```python
from build123d import *
from build123d.topology import SkipClean

# Parameters (mm, degrees)
SKETCH1_W           = 53.05
SKETCH1_H           = 118.2
SKETCH1_W_2         = 45.05
SKETCH1_H_2         = 110.2
BOSS_EXTRUDE1_DEPTH = 60.67
SKETCH2_W           = 53.05
SKETCH2_H           = 118.2
BOSS_EXTRUDE2_DEPTH = 4
SKETCH3_W           = 30
SKETCH3_H           = 22.2
CUT_EXTRUDE1_DEPTH  = 4
SKETCH4_W           = 45
SKETCH4_H           = 38.2
CUT_EXTRUDE2_DEPTH  = 4
SKETCH5_W           = 37.05
SKETCH5_H           = 23
CUT_EXTRUDE3_DEPTH  = 4
SKETCH6_R           = 13.5
SKETCH6_R_2         = 11.5
BOSS_EXTRUDE3_DEPTH = 3.4
SKETCH9_R           = 11.5
CUT_EXTRUDE4_DEPTH  = 5.5
SKETCH10_W          = 1.3
SKETCH10_H          = 30
CUT_EXTRUDE6_DEPTH  = 100.939788873
SKETCH8_R           = 13.5
BOSS_EXTRUDE5_DEPTH = 3
SKETCH12_R          = 3.325
CUT_EXTRUDE8_DEPTH  = 85.508097393


with BuildPart() as part:
    # Sketch1 → Boss-Extrude1 (new body)
    with BuildSketch(Plane.XY):
        Rectangle(SKETCH1_W, SKETCH1_H)
        Rectangle(SKETCH1_W_2, SKETCH1_H_2, mode=Mode.SUBTRACT)
    extrude(amount=BOSS_EXTRUDE1_DEPTH)

    # Sketch2 → Boss-Extrude2 (add)
    with BuildSketch(Plane.XY):
        Rectangle(SKETCH2_W, SKETCH2_H)
    extrude(amount=-BOSS_EXTRUDE2_DEPTH)

    # Sketch3 → Cut-Extrude1 (cut)
    with BuildSketch(Plane(origin=(26.525, 0, 0), x_dir=(0, 0, -1), z_dir=(1, 0, 0))):
        with Locations((-45.67, 0)):
            Rectangle(SKETCH3_W, SKETCH3_H)
    extrude(amount=-CUT_EXTRUDE1_DEPTH, mode=Mode.SUBTRACT)

    # Sketch4 → Cut-Extrude2 (cut)
    with BuildSketch(Plane.ZY.offset(26.525)):
        with Locations((38.17, 0)):
            Rectangle(SKETCH4_W, SKETCH4_H)
    extrude(amount=-CUT_EXTRUDE2_DEPTH, mode=Mode.SUBTRACT)

    # Sketch5 → Cut-Extrude3 (cut)
    with BuildSketch(Plane.XZ.offset(59.1)):
        with Locations((0, 49.17)):
            Rectangle(SKETCH5_W, SKETCH5_H)
    extrude(amount=-CUT_EXTRUDE3_DEPTH, mode=Mode.SUBTRACT)

    # Sketch6 → Boss-Extrude3 (add)
    with BuildSketch(Plane.XY):
        Circle(SKETCH6_R)
        Circle(SKETCH6_R_2, mode=Mode.SUBTRACT)
    extrude(amount=BOSS_EXTRUDE3_DEPTH)

    # Sketch9 → Cut-Extrude4 (cut)
    with SkipClean():  # the faces are left unmerged after this step: merging them gives an invalid solid
        with BuildSketch(Plane(origin=(0, 0, -4), x_dir=(-1, 0, 0), z_dir=(0, 0, -1))):
            Circle(SKETCH9_R)
        extrude(amount=-CUT_EXTRUDE4_DEPTH, mode=Mode.SUBTRACT)
    add(part.part.scale(1), mode=Mode.REPLACE)  # the faces are merged on a copy

    # Sketch10 → Cut-Extrude6 (cut, through all)
    with BuildSketch(Plane(origin=(26.525, 0, 0), x_dir=(0, 0, -1), z_dir=(1, 0, 0))):
        with Locations((3.35, 44.1)):
            Rectangle(SKETCH10_W, SKETCH10_H)
        with Locations((3.35, -44.1)):
            Rectangle(SKETCH10_W, SKETCH10_H)
    extrude(amount=-CUT_EXTRUDE6_DEPTH, mode=Mode.SUBTRACT)

    # Sketch8 → Boss-Extrude5 (add)
    with SkipClean():  # the faces are left unmerged after this step: merging them gives an invalid solid
        with BuildSketch(Plane.XY.offset(3.4)):
            Circle(SKETCH8_R)
        extrude(amount=BOSS_EXTRUDE5_DEPTH)

    # Sketch12 → Cut-Extrude8 (cut, through all)
    with SkipClean():  # the faces are left unmerged after this step: merging them gives an invalid solid
        with BuildSketch(Plane.XY.offset(6.4)):
            Circle(SKETCH12_R)
        extrude(amount=-CUT_EXTRUDE8_DEPTH, mode=Mode.SUBTRACT)


solid = part.part
```
Check sheet for the modelled part. Datum: model origin and axes. Units: mm. A direction names the side the tool comes from. Round coordinates to 2 decimals unless told otherwise and drop trailing zeros. Order: outer loops, then holes, each group sorted by start corner. A loop starts at its lowest first (then second) coordinate and runs counter-clockwise, first axis right, second up. Notation, with made-up numbers: M 84.5,89 L 97.5,89 A28 ccw 97.5,109 Z; hole C 75.5,-39.5 d8. An arc over 180 degrees is marked long. Answer in a Markdown table with one row per item.
(1) Set-up check for faces 1 (the flat face through (18.525, -57, 49)), 2 (the flat face through (25, 0, 30.67)), 3 (the cylindrical face through (-2.93, -13.18, 3.16)): record each of +Z, -Z, +X, -X, +Y, -Y from which the full face is reachable in a straight line by a thin tool's end or side.
Findings:
| item | result |
|---|---|
| face 1 | +Z, -Y |
| face 2 | +Z, +X, -X |
| face 3 | +Z |
(2) Section check B-B on x = 0. Record the boundary of the cut face in (y, z) (3 decimals).
Findings:
| item | result |
|---|---|
| outline | M -59.1,-2.7 L -29.1,-2.7 L -29.1,-4 L -11.5,-4 L -11.5,3.4 L -3.325,3.4 L -3.325,6.4 L -13.5,6.4 L -13.5,0 L -55.1,0 L -55.1,37.67 L -59.1,37.67 Z; M 3.325,3.4 L 11.5,3.4 L 11.5,-4 L 29.1,-4 L 29.1,-2.7 L 59.1,-2.7 L 59.1,60.67 L 55.1,60.67 L 55.1,0 L 13.5,0 L 13.5,6.4 L 3.325,6.4 Z |
(3) Draft check along X on faces 4 (the flat face through (2, 3, 3.4)), 5 (the flat face through (-5, 13, 0)), 6 (the flat face through (0, -59.1, 22)), 7 (the flat face through (-26.525, -1, 14)). Enter one of: +X half, -X half, draft (parallel to the pull), parting line (faces both ways), or undercut.
Findings:
| item | result |
|---|---|
| face 4 | undercut |
| face 5 | undercut |
| face 6 | draft |
| face 7 | -X half |
(4) Section check A-A on z = 54. Record the boundary of the cut face in (x, y) (3 decimals), plus the area to 3 significant figures.
Findings:
| item | result |
|---|---|
| outline | M -26.525,-59.1 L -18.525,-59.1 L -18.525,-55.1 L -22.525,-55.1 L -22.525,-19.1 L -26.525,-19.1 Z; M -26.525,19.1 L -22.525,19.1 L -22.525,55.1 L 22.525,55.1 L 22.525,11.1 L 26.525,11.1 L 26.525,59.1 L -26.525,59.1 Z; M 18.525,-59.1 L 26.525,-59.1 L 26.525,-11.1 L 22.525,-11.1 L 22.525,-55.1 L 18.525,-55.1 Z |
| area | 916 mm^2 |
(5) Material ranges on line 1 along Y through (x, z) = (0, 4.6) (3 decimals); line 2 along Y through (x, z) = (0, 2.15); line 3 along X through (y, z) = (-25.5, 14.5) (3 decimals), recorded low to high. Write a range as from..to.
Findings:
| item | result |
|---|---|
| line 1 | y = -59.1..-55.1, -13.5..-3.325, 3.325..13.5, 55.1..59.1 |
| line 2 | y = -59.1..-55.1, -13.5..-11.5, 11.5..13.5, 55.1..59.1 |
| line 3 | x = -26.525..-22.525, 22.525..26.525 |
(6) Gauge pin test, flat ends, axial feed: pin 1 (2 mm diameter, centred on x = 25, y = -4.5, fed in from +Z); pin 2 (4.5 mm diameter, centred on x = -24.5, y = -9.5, fed in from +Z); pin 3 (9 mm diameter, centred on x = 0, y = 44.5, fed in from -Z). Record the tip position at first contact, or that the pin passes through.
Findings:
| item | result |
|---|---|
| pin 1 | stops at z = 30.67 |
| pin 2 | stops at z = 15.67 |
| pin 3 | stops at z = -2.7 |
(7) Section check D-D on z = 28. Record the boundary of the cut face in (x, y) (3 decimals), plus the area to 3 significant figures.
Findings:
| item | result |
|---|---|
| outline | M -26.525,-59.1 L 26.525,-59.1 L 26.525,59.1 L -26.525,59.1 L -26.525,19.1 L -22.525,19.1 L -22.525,55.1 L 22.525,55.1 L 22.525,-55.1 L -22.525,-55.1 L -22.525,-19.1 L -26.525,-19.1 Z |
| area | 1,150 mm^2 |
(8) Section check C-C on z = 35. Record the boundary of the cut face in (x, y) (3 decimals), plus the area to 3 significant figures.
Findings:
| item | result |
|---|---|
| outline | M -26.525,-59.1 L 26.525,-59.1 L 26.525,-11.1 L 22.525,-11.1 L 22.525,-55.1 L -22.525,-55.1 L -22.525,-19.1 L -26.525,-19.1 Z; M -26.525,19.1 L -22.525,19.1 L -22.525,55.1 L 22.525,55.1 L 22.525,11.1 L 26.525,11.1 L 26.525,59.1 L -26.525,59.1 Z |
| area | 1,060 mm^2 |
